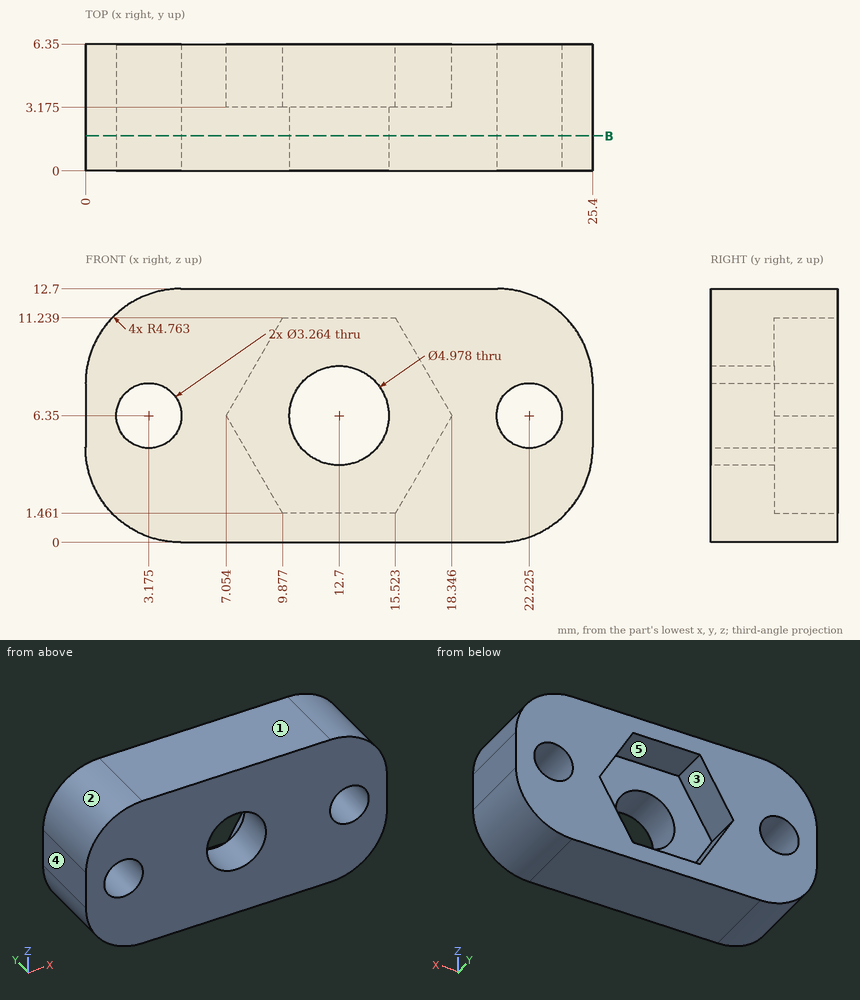
Check sheet for the drawn part. Datum: minimum x, y, z corner. Units: mm. A direction names the side the tool comes from. Coordinates: 2 decimals unless noted, no trailing zeros. Answer in a Markdown table with one row per item.
1. Access from +Z, -Z, +X, -X, +Y, -Y to the whole of each face (thin tool, end or side, straight path). Record for the marked faces 4 and 5.
Check values:
| item | result |
|---|---|
| face 4 | +Z, -Z, -X, +Y, -Y |
| face 5 | +Y |
2. Go/stop test with a flat-tipped pin: pin 1 (2 mm diameter, centred on x = 2.5, y = 3.5, fed in from +Z). Record where the tip stops, or that it passes through.
Check values:
| item | result |
|---|---|
| pin 1 | stops at z = 12.53 |
3. Release check for a two-part mould opening along X. For the marked faces 1, 2 and 3 record: released by +X, released by -X, zero draft, split by the parting line, or undercut.
Check values:
| item | result |
|---|---|
| face 1 | zero draft |
| face 2 | released by -X |
| face 3 | undercut |
4. Material ranges on line 1 along X through (y, z) = (1.95, 6.35); line 2 along X through (y, z) = (2, 5.25) (1 decimal); line 3 along Z through (x, y) = (12.25, 5.5), recorded low to high. Write a range as [from, to].
Check values:
| item | result |
|---|---|
| line 1 | x = [0, 1.54], [4.81, 10.21], [15.19, 20.59], [23.86, 25.4] |
| line 2 | x = [0, 2], [4.4, 10.5], [14.9, 21], [23.4, 25.4] |
| line 3 | z = [0, 1.46], [11.24, 12.7] |
5. Sectioned sample at B-B, the plane y = 1.75. Give the number of separate pieces and of enclosed holes in the cut face, then the cut area to 3 significant figures.
Check values:
| item | result |
|---|---|
| separate pieces | 1 |
| enclosed holes | 3 |
| area | 267 mm2 |
